from build123d import *

# Parameters (mm, degrees)
SKETCH1_W           = 118
SKETCH1_H           = 78
MAIN_BOX_UP_DEPTH   = 34
SKETCH2_W           = 112
SKETCH2_H           = 72
MAIN_BOX_INTO_DEPTH = 32
SKETCH4_R           = 1.4
SKETCH4_W           = 12
SKETCH4_H           = 12
GPS_DEPTH           = 3
SKETCH5_R           = 2.25
SKETCH5_R_2         = 3.6
CUT_EXTRUDE3_DEPTH  = 3
SKETCH6_R           = 0.85
CUT_EXTRUDE4_DEPTH  = 4


with BuildPart() as part:
    # Sketch1 → Main Box Up (new body)
    with BuildSketch(Plane(origin=(0, 0, 0), x_dir=(1, 0, 0), z_dir=(0, 1, 0))):
        Rectangle(SKETCH1_W, SKETCH1_H)
    extrude(amount=MAIN_BOX_UP_DEPTH)

    # Sketch2 → Main Box Into (cut)
    with BuildSketch(Plane(origin=(0, 34, 0), x_dir=(1, 0, 0), z_dir=(0, 1, 0))):
        Rectangle(SKETCH2_W, SKETCH2_H)
    extrude(amount=-MAIN_BOX_INTO_DEPTH, mode=Mode.SUBTRACT)

    # Sketch4 → GPS (cut)
    with BuildSketch(Plane.ZY.offset(-56)):
        with Locations((-30.16, 28.16)):
            Circle(SKETCH4_R)
        with Locations((-9.84, 28.16)):
            Circle(SKETCH4_R)
        with Locations((-30.16, 7.84)):
            Circle(SKETCH4_R)
        with Locations((-9.84, 7.84)):
            Circle(SKETCH4_R)
        with Locations((-20, 18)):
            Rectangle(SKETCH4_W, SKETCH4_H)
    extrude(amount=-GPS_DEPTH, mode=Mode.SUBTRACT)

    # Sketch5 → Cut-Extrude3 (cut)
    with BuildSketch(Plane.ZY.offset(-56)):
        with Locations((12.14, 28.16)):
            Circle(SKETCH5_R)
        with Locations((32.46, 28.16)):
            Circle(SKETCH5_R)
        with Locations((12.14, 7.84)):
            Circle(SKETCH5_R)
        with Locations((32.46, 7.84)):
            Circle(SKETCH5_R)
        with Locations((22.3, 18)):
            Circle(SKETCH5_R_2)
    extrude(amount=-CUT_EXTRUDE3_DEPTH, mode=Mode.SUBTRACT)

    # Sketch6 → Cut-Extrude4 (cut)
    with BuildSketch(Plane(origin=(0, 34, 0), x_dir=(1, 0, 0), z_dir=(0, 1, 0))):
        with Locations(Location((-57.5, 37.5, 0), (0, 0, 270))):
            Circle(SKETCH6_R)
        with Locations(Location((-57.5, -37.5, 0), (0, 0, 270))):
            Circle(SKETCH6_R)
        with Locations(Location((57.5, -37.5, 0), (0, 0, 270))):
            Circle(SKETCH6_R)
        with Locations(Location((57.5, 37.5, 0), (0, 0, 270))):
            Circle(SKETCH6_R)
        with Locations(Location((0, 37.5, 0), (0, 0, 270))):
            Circle(SKETCH6_R)
        with Locations(Location((0, -37.5, 0), (0, 0, 270))):
            Circle(SKETCH6_R)
    extrude(amount=-CUT_EXTRUDE4_DEPTH, mode=Mode.SUBTRACT)


solid = part.part
Geometry: final body of the model. Coordinates: model frame, mm. A direction names the side the tool comes from. Coordinates: 2 decimals unless noted, no trailing zeros. Order: outer loops, then holes, each group sorted by start corner. A loop starts at its lowest first (then second) coordinate and runs counter-clockwise, first axis right, second up. Notation, with made-up numbers: M -7.75,76.5 L 22.25,76.5 A23 ccw 22.25,109.5 Z; hole C -23.5,43.5 d5. An arc over 180 degrees is marked long. One line per question, with ' | ' between items. Start each with the question number.
Item 1: Cut plane D-D, the plane y = 18. Return the cut outline in (x, z), then the cut area to 3 significant figures.
Item 2: Ray query, probe 1 along Z at (x, y) = (-57.5, 31.3); probe 2 along Y at (x, z) = (58.1, -9.84); probe 3 along X at (y, z) = (28, 2.5). Return the intervals inside material, ascending. Write a range as [from, to].
Item 3: Cut plane C-C, the plane z = 7. Return the cut outline in (x, y).
Item 4: Draft query along Y for faces 4 (the flat face through (-59, 17, 1)), 5 (the flat face through (57, 12, -20)). Return one class per face: released by +Y, released by -Y, zero draft, split by the parting line, or undercut.
Item 5: Cut plane B-B, the plane x = -35.5. Return the cut outline in (y, z), then the cut area to 3 significant figures.
Item 6: Cut plane A-A, the plane y = 7.84. Return the cut outline in (x, z), then the cut area to 3 significant figures.
Item 7: Pin query (flat end, axial travel): pin 1 Ø0.5 at (x, z) = (-57.5, 37.5) entering from +Y; pin 2 Ø3.5 at (y, z) = (7.84, 12.14) entering from +X; pin 3 Ø4 at (x, z) = (-6.5, -8.5) entering from +Y. Return the tip coordinate at first contact, or that it passes through.
Item 8: Set-up query: faces 1 (the cylindrical face through (57.48, 26.92, -29.51)), 2 (the flat face through (56, 18, 1)), 3 (the flat face through (59, 17, 1)). Return all of +Z, -Z, +X, -X, +Y, -Y with unobstructed straight access to the full face (end or side cutting, diameter ignored); none if empty.
A:
1) outline: M -59,-39 L 59,-39 L 59,-26 L 56,-26 L 56,-36 L -56,-36 L -56,36 L 56,36 L 56,25.9 L 59,25.9 L 59,39 L -59,39 Z; M 56,-14 L 59,-14 L 59,18.7 L 56,18.7 Z | area: 1,080 mm2
2) probe 1: z = [-39, -38.35], [-36.65, 36.65], [38.35, 39] | probe 2: y = [0, 6.44], [9.24, 26.76], [29.56, 34] | probe 3: x = [-59, -56], [56, 59]
3) outline: M -59,0 L 59,0 L 59,34 L 56,34 L 56,2 L -56,2 L -56,34 L -59,34 Z
4) face 4: zero draft | face 5: undercut
5) outline: M 0,-39 L 34,-39 L 34,-36 L 2,-36 L 2,36 L 34,36 L 34,39 L 0,39 Z | area: 348 mm2
6) outline: M -59,-39 L 59,-39 L 59,-31.56 L 56,-31.56 L 56,-36 L -56,-36 L -56,36 L 56,36 L 56,34.71 L 59,34.71 L 59,39 L -59,39 Z; M 56,-28.76 L 59,-28.76 L 59,-11.24 L 56,-11.24 Z; M 56,-8.44 L 59,-8.44 L 59,9.89 L 56,9.89 Z; M 56,14.39 L 59,14.39 L 59,30.21 L 56,30.21 Z | area: 1,100 mm2
7) pin 1: stops at y = 30 | pin 2: stops at x = -56 | pin 3: stops at y = 2
8) face 1: +X | face 2: +Y | face 3: +Z, -Z, +X, +Y, -Y
